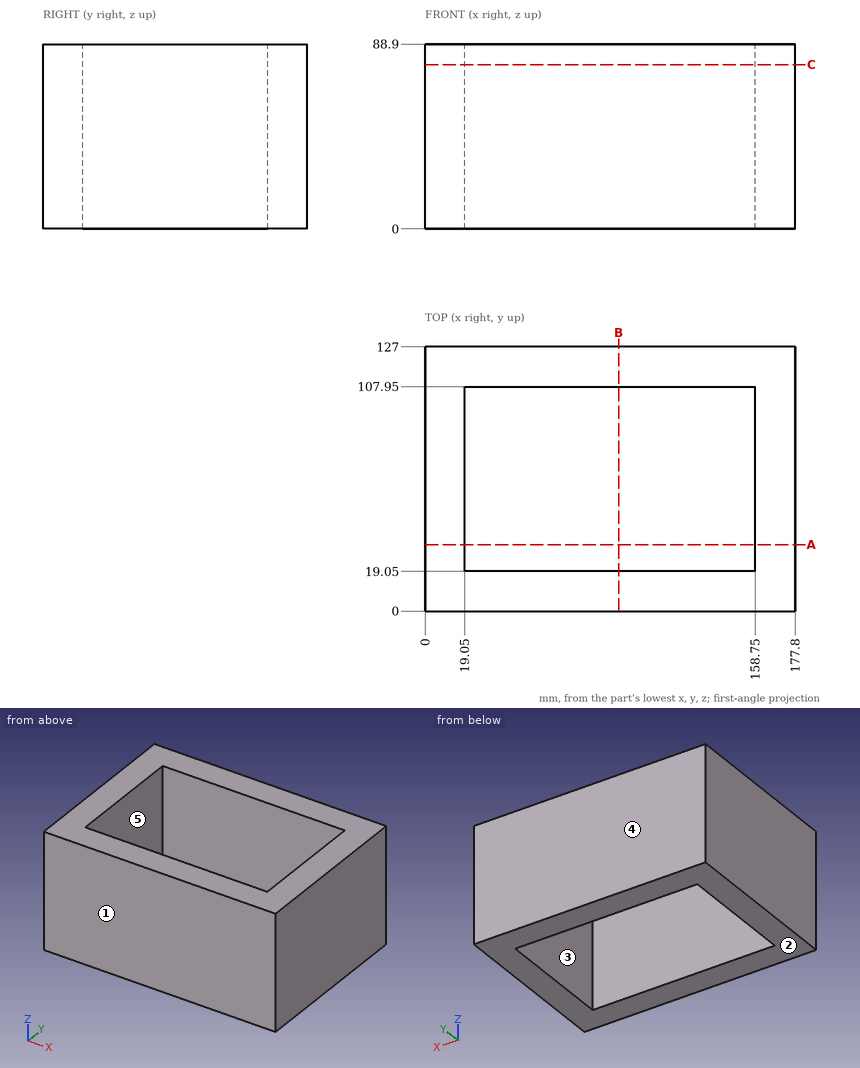
For this review, use the dimensioned drawing (mm, ordinates from the lowest corner) and the shaded views. A direction names the side the tool comes from. Round coordinates to 2 decimals unless told otherwise and drop trailing zeros. Write each loop counter-clockwise with the first axis right and the second up, starting at its lowest first coordinate (ties: lowest second). Pieces come first, ordered by that corner, then holes. Notation, with made-up numbers: (84, 89.25) -> (92, 89.25) arc R26 ccw to (92, 119.25) -> close; hole circle Ø11 at (-28, 3.5). An arc over 180 degrees is marked (long way). One line per item, written item: value. Start each with the question number.
Q1. To check wall thickness, follow probe 1 along X at (y, z) = (94.5, 32); probe 2 along Y at (x, z) = (83, 82). State the ranges of each line that lie inside material, in increasing order.
Q2. Insertion check: P1, Ø10, axis at x = 152.5, y = 14.5, coming from the -Z side. The pin has a flat end and moves straight along its axis. Give the tip position at first contact, or say it passes through.
Q3. Add section C-C (z = 79). Give the boundary of the cut face in (x, y), then the cut area to 3 significant figures.
Q4. Add section A-A (y = 32). Give the boundary of the cut face in (x, z).
Q5. Tool access review of the marked faces 4 and 5: name each direction out of +Z, -Z, +X, -X, +Y, -Y from which nothing blocks a thin tool from reaching the whole face with its end or side.
Q6. Add section B-B (x = 93). Give the boundary of the cut face in (y, z).
Q7. The part is to be moulded in two halves that separate along Y. For the marked faces 1, 2 and 3, say which applies: pulls with the +Y half, pulls with the -Y half, needs draft (parallel to the pull), parting line crosses it, or undercut.
Response:
1. probe 1: x = 0 to 19.05, 158.75 to 177.8
1. probe 2: y = 0 to 19.05, 107.95 to 127
2. P1: stops at z = 0
3. outline: (0, 0) -> (177.8, 0) -> (177.8, 127) -> (0, 127) -> close; hole (19.05, 19.05) -> (158.75, 19.05) -> (158.75, 107.95) -> (19.05, 107.95) -> close
3. area: 10,200 mm^2
4. outline: (0, 0) -> (19.05, 0) -> (19.05, 88.9) -> (0, 88.9) -> close; (158.75, 0) -> (177.8, 0) -> (177.8, 88.9) -> (158.75, 88.9) -> close
5. face 4: +Z, -Z, +X, -X, +Y
5. face 5: +Z, -Z
6. outline: (0, 0) -> (19.05, 0) -> (19.05, 88.9) -> (0, 88.9) -> close; (107.95, 0) -> (127, 0) -> (127, 88.9) -> (107.95, 88.9) -> close
7. face 1: pulls with the -Y half
7. face 2: needs draft
7. face 3: undercut
